Design review of the part built by this model. Coordinates are the model's own, in mm. A direction names the side the tool comes from. Coordinates: 2 decimals unless noted, no trailing zeros. Write each loop counter-clockwise with the first axis right and the second up, starting at its lowest first coordinate (ties: lowest second). Pieces come first, ordered by that corner, then holes. Notation, with made-up numbers: (72.25, -19) -> (126.25, -19) arc R20 ccw to (126.25, 18) -> close; hole circle Ø9 at (-2.75, -2.75). An arc over 180 degrees is marked (long way). Answer in a Markdown table with one row per item. Add a question column.
Item 1: Draft analysis for pull direction Z (two halves, no side actions). For faces 1 (the face through (0, 14, 3)), 2 (the face through (3, 49, 0)), 3 (the face through (5, 14, 6.5)), 4 (the face through (5, 12, 2.5)), state which applies: released by +Z, released by -Z, zero draft, split by the parting line, or undercut.
Item 2: Take a section at B-B, the plane z = 0. Write out the cut boundary in (x, y), and give its area (3 significant figures).
Item 3: For faces 5 (the face through (2.7, 24, 0.1)), 6 (the face through (5.675, 8, 4)), 7 (the face through (5, 12, -2.5)), 8 (the face through (8, 1, 5)), 9 (the face through (1, 2, -4)), list the 3-axis set-ups (+Z, -Z, +X, -X, +Y, -Y) from which the entire face can be reached by the end or side of a thin tool; tool diameter is ignored.
Item 4: Take a section at C-C, the plane x = 1.5. Write out the cut boundary in (y, z), and give its area (3 significant figures).
Item 5: Clearance check with flat-ended pins moving along their axes: P1, Ø5, axis at x = 5, y = 5, coming from the -Z side; P2, Ø5, axis at x = 2, z = 2.5, coming from the +Y side; P3, Ø1, axis at x = 8, z = 2, coming from the +Y side; P4, Ø1.5, axis at y = 8.5, z = -5, coming from the +X side. State where each tip first meets the part, or that it passes through.
Item 6: To check wall thickness, follow line 1 (Y direction, x = 5, z = -3.3); line 2 (Z direction, x = 5.25, y = 10.5); line 3 (X direction, y = 5, z = 4.95). State the ranges of each line that lie inside material, in increasing order.
Item 7: Take a section at D-D, the plane y = 35. Write out the cut boundary in (x, z), and give its area (3 significant figures).
Item 8: Take a section at A-A, the plane y = 17. Write out the cut boundary in (x, z).
Autodesk Inventor part; units mm, degrees
ref_plane "YZ Plane" through (0, 0, 0) normal (1, 0, 0) x (0, 1, 0)
ref_plane "XZ Plane" through (0, 0, 0) normal (0, 1, 0) x (-1, 0, 0)
ref_plane "XY Plane" through (0, 0, 0) normal (0, 0, 1) x (1, 0, 0)
sketch "Sketch1" plane through (0, 0, 0) normal (1, 0, 0) x (0, 1, 0)
  line L0 (0, 6.5) -> (24, 6.5)
  line L1 (24, 6.5) -> (24, -6.5)
  line L2 (24, -6.5) -> (0, -6.5)
  line L3 (0, -6.5) -> (0, -2.5)
  line L4 (0, -2.5) -> (20, -2.5)
  line L5 (20, -2.5) -> (20, 2.5)
  line L6 (20, 2.5) -> (0, 2.5)
  line L7 (0, 2.5) -> (0, 6.5)
  point P0 (0, 0)
  dimension "d0" = 4
  dimension "d1" = 20
  dimension "d2" = 4
  dimension "d3" = 5
  dimension "d11" = 2.5
  dimension "d12" = 0
extrude "Extrusion1" add sketch "Sketch1" along normal blind 10
sketch "Sketch2" plane through (0, 24, 6.5) normal (0, 1, 0) x (1, 0, 0)
  circle A0 centre (5, 6.5) radius 2
  line L0 (0, 0) -> (0, 13)
  line L1 (0, 13) -> (10, 13)
  point P0 (0, 6.5)
  dimension "d6" = 4
  dimension "d7" = 5
  dimension "d8" = 6.5
extrude "Extrusion2" add sketch "Sketch2" along normal blind 50
sketch "Sketch3" plane through (0, 0, 0) normal (0, 0, 1) x (1, 0, 0)
  line L0 (7, 74) -> (3, 74)
  line L1 (3, 74) -> (5, 74)
  line L2 (5, 74) -> (5, 84)
  arc A0 (5, 84) -> (3, 74) centre (5, 78.8) ccw
  point P0 (0, 0)
  dimension "d13" = 10
revolve "Revolution1" add sketch "Sketch3" angle 360 about axis through (5, 74, 0) along (0, 1, 0)
fillet "Fillet1" radius 5 4 edges at (0, 0, -4.5) (10, 0, -4.5) (10, 0, 4.5) (0, 0, 4.5)
hole "Hole1" at (5, 5, -6.5) direction (0, 0, 1) diameter 5.5 end through all
sketch "Sketch4" plane through (10, 24, -6.5) normal (0, 0, -1) x (-1, 0, 0)
  circle A0 centre (5, -19) radius 2.75
  line L0 (4.325, -16.3341) -> (4.325, -14.9841)
  line L1 (4.325, -14.9841) -> (5.675, -14.9841)
  line L2 (5.675, -14.9841) -> (5.675, -16.3341)
  line L3 (4.325, -16.3341) -> (5.675, -16.3341)
  point P0 (10, -24)
  dimension "d25" = 1.35
  dimension "d26" = 0.675
  dimension "d27" = 1.35
extrude "Extrusion3" cut sketch "Sketch4" against normal through all contours A0 L0 L1 L2
properties part number "EndJoint"
Answers:
| question | item | result |
|---|---|---|
| 1 | face 1 | zero draft |
| 1 | face 2 | split by the parting line |
| 1 | face 3 | released by +Z |
| 1 | face 4 | undercut |
| 2 | outline | (0, 20) -> (10, 20) -> (10, 24) -> (7, 24) -> (7, 74) arc R5.2 ccw (long way) to (3, 74) -> (3, 24) -> (0, 24) -> close |
| 2 | area | 324 mm^2 |
| 3 | face 5 | none |
| 3 | face 6 | +Z, -Z |
| 3 | face 7 | +X, -X, -Y |
| 3 | face 8 | +Z, -Z, +X, -Y |
| 3 | face 9 | +Z, -Z, -X, -Y |
| 4 | outline | (1.43, -6.5) -> (24, -6.5) -> (24, 6.5) -> (1.43, 6.5) -> (1.43, 2.5) -> (20, 2.5) -> (20, -2.5) -> (1.43, -2.5) -> close; circle Ø7.69 at (78.8, 0) |
| 4 | area | 247 mm^2 |
| 5 | P1 | passes through |
| 5 | P2 | stops at y = 83.81 |
| 5 | P3 | stops at y = 82.97 |
| 5 | P4 | stops at x = 10 |
| 6 | line 1 | y = 0 to 2.25, 9.02 to 24, 74.78 to 82.82 |
| 6 | line 2 | z = -6.5 to -2.5, 2.5 to 6.5 |
| 6 | line 3 | x = 0 to 2.25, 7.75 to 10 |
| 7 | outline | circle Ø4 at (5, 0) |
| 7 | area | 12.6 mm^2 |
| 8 | outline | (0, -6.5) -> (10, -6.5) -> (10, -2.5) -> (0, -2.5) -> close; (0, 2.5) -> (10, 2.5) -> (10, 6.5) -> (0, 6.5) -> close |
